Verification items for the finished model (mm, model axes). Face numbers are marked on the shaded views. A direction names the side the tool comes from. Round coordinates to 2 decimals unless told otherwise and drop trailing zeros. Loops run counter-clockwise (first coordinate to the right, second up) from the corner with the lowest first, then second, coordinate; pieces in that order, holes last. Notation, with made-up numbers: (-34, -18.5) - (25, -18.5) arc R8 ccw to (25, -10.5) - close; hole circle Ø8 at (88, 46.25). An arc over 180 degrees is marked (long way). Use CSV: the item, a comma, the result in double quotes.
```python
from build123d import *

# Parameters (mm, degrees)
SKETCH1_R           = 11.5
BOSS_EXTRUDE1_DEPTH = 6.5
SKETCH2_R           = 5
BOSS_EXTRUDE2_DEPTH = 0.5
SKETCH3_R           = 4
BOSS_EXTRUDE3_DEPTH = 5
SKETCH4_R           = 6.5
CUT_EXTRUDE1_DEPTH  = 4
SKETCH5_R           = 5.5
CUT_EXTRUDE2_DEPTH  = 0.5
SKETCH6_R           = 1.75
CUT_EXTRUDE3_DEPTH  = 7.5
SKETCH7_R           = 1.6
CUT_EXTRUDE4_DEPTH  = 6.5
SKETCH8_R           = 2
CUT_EXTRUDE5_DEPTH  = 4
CIRPATTERN1_COUNT   = 6
CHAMFER2_SIZE       = 0.5


with BuildPart() as part:
    # Sketch1 → Boss-Extrude1 (new body)
    with BuildSketch(Plane(origin=(0, 0, 0), x_dir=(1, 0, 0), z_dir=(0, 1, 0))):
        with Locations(Location((0, 0, 0), (0, 0, 90))):
            Circle(SKETCH1_R)
    extrude(amount=BOSS_EXTRUDE1_DEPTH)

    # Sketch2 → Boss-Extrude2 (add)
    with BuildSketch(Plane.XZ):
        with Locations(Location((0, 0, 0), (0, 0, 270))):
            Circle(SKETCH2_R)
    extrude(amount=BOSS_EXTRUDE2_DEPTH)

    # Sketch3 → Boss-Extrude3 (add)
    with BuildSketch(Plane.XZ.offset(0.5)):
        with Locations(Location((0, 0, 0), (0, 0, 270))):
            Circle(SKETCH3_R)
    extrude(amount=BOSS_EXTRUDE3_DEPTH)

    # Sketch4 → Cut-Extrude1 (cut)
    with BuildSketch(Plane(origin=(0, 6.5, 0), x_dir=(1, 0, 0), z_dir=(0, 1, 0))):
        with Locations(Location((0, 0, 0), (0, 0, 270))):
            Circle(SKETCH4_R)
    extrude(amount=-CUT_EXTRUDE1_DEPTH, mode=Mode.SUBTRACT)

    # Sketch5 → Cut-Extrude2 (cut)
    with BuildSketch(Plane(origin=(0, 2.5, 0), x_dir=(1, 0, 0), z_dir=(0, 1, 0))):
        with Locations(Location((0, 0, 0), (0, 0, 270))):
            Circle(SKETCH5_R)
    extrude(amount=-CUT_EXTRUDE2_DEPTH, mode=Mode.SUBTRACT)

    # Sketch6 → Cut-Extrude3 (cut)
    with BuildSketch(Plane(origin=(0, 2, 0), x_dir=(1, 0, 0), z_dir=(0, 1, 0))):
        with Locations(Location((0, 0, 0), (0, 0, 270))):
            Circle(SKETCH6_R)
    extrude(amount=-CUT_EXTRUDE3_DEPTH, mode=Mode.SUBTRACT)

    # Sketch7 → Cut-Extrude4 (cut)
    with BuildSketch(Plane(origin=(0, 6.5, 0), x_dir=(1, 0, 0), z_dir=(0, 1, 0))):
        with Locations(Location((0, 9, 0), (0, 0, 270))):
            Circle(SKETCH7_R)
    cut_extrude4 = extrude(amount=-CUT_EXTRUDE4_DEPTH, mode=Mode.SUBTRACT)

    # Sketch8 → Cut-Extrude5 (cut)
    with BuildSketch(Plane.XZ):
        with Locations(Location((0, -9, 0), (0, 0, 270))):
            Circle(SKETCH8_R)
    cut_extrude5 = extrude(amount=-CUT_EXTRUDE5_DEPTH, mode=Mode.SUBTRACT)

    # CirPattern1: Cut-Extrude4, Cut-Extrude5 ×6 about axis
    cirpattern1_axis = Axis((0, 0, 0), (0, 1, 0))
    add([cut_extrude4.rotate(cirpattern1_axis, i * 360 / CIRPATTERN1_COUNT) for i in range(1, CIRPATTERN1_COUNT)], mode=Mode.SUBTRACT)
    add([cut_extrude5.rotate(cirpattern1_axis, i * 360 / CIRPATTERN1_COUNT) for i in range(1, CIRPATTERN1_COUNT)], mode=Mode.SUBTRACT)

    # Chamfer2
    chamfer2_edges = [part.edges().sort_by_distance(p)[0] for p in [
        (0, -5.5, 4),
        (0, 6.5, -6.5),
        (0, 0, 11.5),
        (0, 2, -1.75),
        (0, -5.5, -1.75),
        (0, 6.5, 11.5),
    ]]
    chamfer(chamfer2_edges, length=CHAMFER2_SIZE - 0.0001)  # a hair under: the kernel refuses the full size


solid = part.part
```
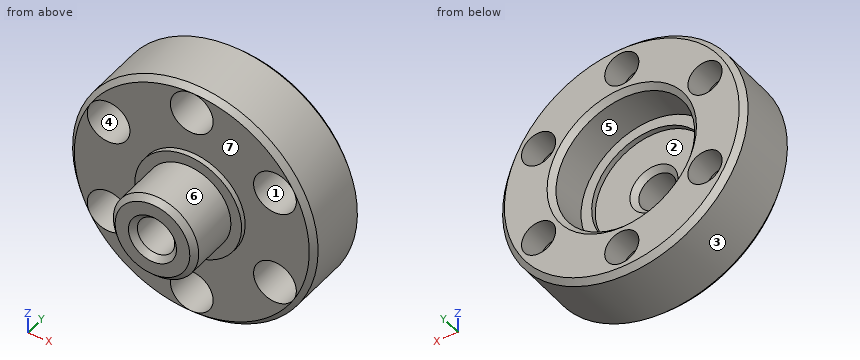
1) Access from +Z, -Z, +X, -X, +Y, -Y to the whole of each face (thin tool, end or side, straight path). Record for the marked faces 1, 2 and 3.
Returned:
face 1,"-Y"
face 2,"+Y"
face 3,"+Y, -Y"
2) Gauge pin test, flat ends, axial feed: pin 1 Ø6 at (y, z) = (0, 2) entering from +X; pin 2 Ø1 at (y, z) = (-3.5, 1) entering from +X; pin 3 Ø3 at (x, z) = (-7.5, -5.5) entering from -Y; pin 4 Ø1.9 at (x, z) = (0, -9) entering from -Y. Record the tip position at first contact, or that the pin passes through.
Returned:
pin 1,"stops at x = 11.5"
pin 2,"stops at x = 3.97"
pin 3,"stops at y = 0"
pin 4,"passes through"
3) Mould release check, pull along X, two halves, no side actions. Record for the marked faces 4, 5, 6 and 7: +X half, -X half, draft (parallel to the pull), parting line (faces both ways), or undercut.
Returned:
face 4,"undercut"
face 5,"undercut"
face 6,"parting line"
face 7,"draft"
4) Cross-section at A-A, the plane y = 3. Record the cut outline in (x, z), then the cut area to 3 significant figures.
Returned:
outline,"circle Ø23 at (0, 0); hole circle Ø4 at (-7.79, -4.5); hole circle Ø4 at (-7.79, 4.5); hole circle Ø13 at (0, 0); hole circle Ø4 at (0, -9); hole circle Ø4 at (0, 9); hole circle Ø4 at (7.79, -4.5); hole circle Ø4 at (7.79, 4.5)"
area,"207 mm²"
5) Thickness scan on probe 1 along X at (y, z) = (-2.75, 0); probe 2 along X at (y, z) = (4.65, 4.5); probe 3 along X at (y, z) = (3.9, 0). Record the ranges inside material, lowest first. Write a range as [from, to].
Returned:
probe 1,"x = [-4, -1.75], [1.75, 4]"
probe 2,"x = [-10.58, -9.39], [-6.19, -4.69], [4.69, 6.19], [9.39, 10.58]"
probe 3,"x = [-11.5, -6.5], [6.5, 11.5]"
6) Cross-section at C-C, the plane y = -3.5. Record the cut outline in (x, z).
Returned:
outline,"circle Ø8 at (0, 0); hole circle Ø3.5 at (0, 0)"
7) Cross-section at B-B, the plane x = 0. Count the separate pieces of the cut face and the enclosed holes in it, then the cut area to 3 significant figures.
Returned:
separate pieces,"4"
enclosed holes,"0"
area,"61.3 mm²"
